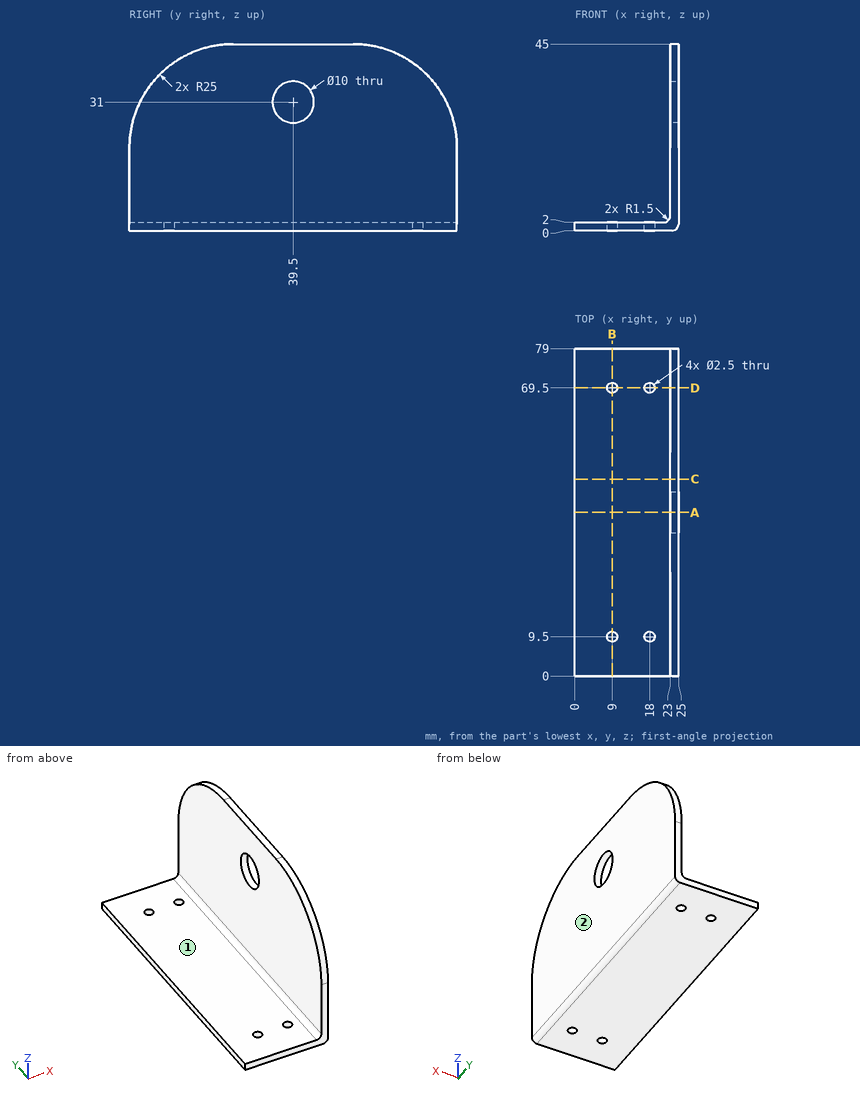
Input: dimensioned drawing with shaded views. Units: mm. Origin: part minimum x, y, z. A direction names the side the tool comes from. Give positions to 0.01 mm unless a question says otherwise; leave off trailing zeros. Write each loop counter-clockwise with the first axis right and the second up, starting at its lowest first coordinate (ties: lowest second). Pieces come first, ordered by that corner, then holes.
1. Section query B-B (x = 9). Return the cut outline in (y, z), then the cut area to 3 significant figures.
2. Section query D-D (y = 69.5). Return the cut outline in (x, z).
3. Section query A-A (y = 39.5). Return the cut outline in (x, z), then the cut area to 3 significant figures.
4. Section query C-C (y = 47.5). Return the cut outline in (x, z).
5. First-contact query: pin 1 (5 mm diameter, centred on x = 21.5, z = 34, fed in from -Y); pin 2 (12.5 mm diameter, centred on y = 42, z = 26, fed in from -X); pin 3 (1.5 mm diameter, centred on x = 17.5, y = 71, fed in from +Z). Flat tips, straight axial feed; report the tip coordinate or a pass-through.
6. Access query for the marked faces 1 and 2. Directions: +Z, -Z, +X, -X, +Y, -Y. A direction counts if a zero-diameter tool reaches every point of the face in a straight line with its end or side. Return the directions, or none.
7. Material intervals for line 1 along Y through (x, z) = (18, 0.85); line 2 along Z through (x, y) = (10, 29); line 3 along X through (y, z) = (71, 27.5), sorted ascending.
Output values:
1. outline: (0, 0) - (8.25, 0) - (8.25, 2) - (0, 2) - close; (10.75, 0) - (68.25, 0) - (68.25, 2) - (10.75, 2) - close; (70.75, 0) - (79, 0) - (79, 2) - (70.75, 2) - close
1. area: 148 mm2
2. outline: (0, 0) - (7.75, 0) - (7.75, 2) - (0, 2) - close; (10.25, 0) - (16.75, 0) - (16.75, 2) - (10.25, 2) - close; (19.25, 0) - (23.5, 0) arc R1.5 ccw to (25, 1.5) - (25, 39.62) - (23, 39.62) - (23, 3.5) arc R1.5 cw to (21.5, 2) - (19.25, 2) - close
3. outline: (0, 0) - (23.5, 0) arc R1.5 ccw to (25, 1.5) - (25, 26) - (23, 26) - (23, 3.5) arc R1.5 cw to (21.5, 2) - (0, 2) - close; (23, 36) - (25, 36) - (25, 45) - (23, 45) - close
3. area: 116 mm2
4. outline: (0, 0) - (23.5, 0) arc R1.5 ccw to (25, 1.5) - (25, 45) - (23, 45) - (23, 3.5) arc R1.5 cw to (21.5, 2) - (0, 2) - close
5. pin 1: stops at y = 3.07
5. pin 2: stops at x = 23
5. pin 3: stops at z = 2
6. face 1: +Z, -X, +Y, -Y
6. face 2: +Z, -Z, +X, +Y, -Y
7. line 1: y = 0 to 8.25, 10.75 to 68.25, 70.75 to 79
7. line 2: z = 0 to 2
7. line 3: x = 23 to 25
